Could you check a few things on this drawing? It's one solid part, dimensions in mm from its lowest x, y, z. Give positions to 0.01 mm unless a question says otherwise; leave off trailing zeros. Order: outer loops, then holes, each group sorted by start corner. A loop starts at its lowest first (then second) coordinate and runs counter-clockwise, first axis right, second up. Notation, with made-up numbers: M 65.25,6.25 L 85.25,6.25 A13 ccw 85.25,28.25 Z; hole C -23.75,42.5 d11. An arc over 180 degrees is marked long. Use one line per item in the form item = value. Start each with the question number.
1. We'd pull the mould along X, two halves only. Please class the marked faces 1, 2 and 3: +X half, -X half, draft (parallel to the pull), parting line (faces both ways), or undercut.
2. I want a section at C-C, the plane y = 2.25. List the corners of the cut face in (x, z) for me (3 decimals), and give its area (3 significant figures).
3. Will these pins go through, and if not, where does the flat tip stop? P1, Ø2, axis at x = 18.5, z = 49, coming from the -Y side; P2, Ø3, axis at x = 15, y = 4, coming from the -Z side.
4. I want a section at A-A, the plane z = 26.5. List the corners of the cut face in (x, y) for me.
5. I need wall thicknesses on L1, parallel to X at y = 1.75, z = 21.5; L2, parallel to Z at x = 12, y = 2; L3, parallel to Y at x = 14, z = 32. Which ranges of each line are inside material? Lowest first, please.
6. I want a section at B-B, the plane x = 10. List the corners of the cut face in (y, z) for me (3 decimals), and give its area (3 significant figures).
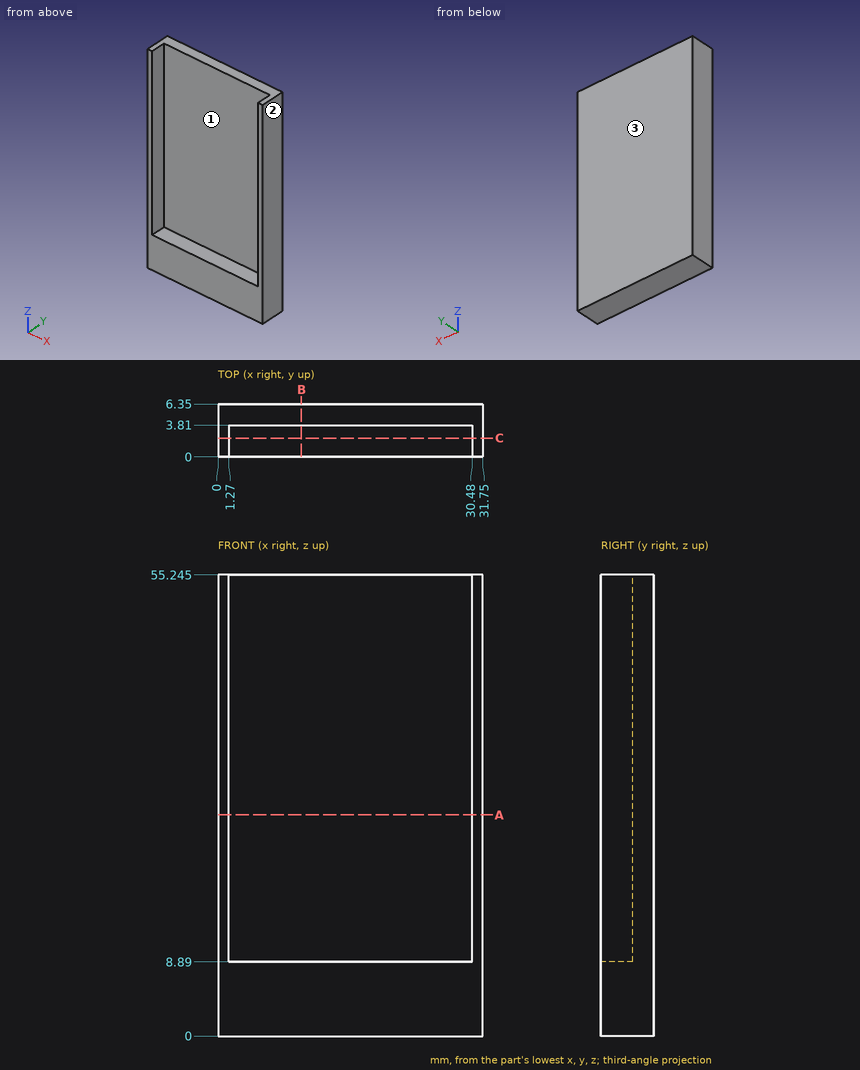
Check result:
q1.face_1 = undercut
q1.face_2 = +X half
q1.face_3 = draft
q2.outline = M 0,0 L 31.75,0 L 31.75,55.245 L 30.48,55.245 L 30.48,8.89 L 1.27,8.89 L 1.27,55.245 L 0,55.245 Z
q2.area = 400 mm2
q3.P1 = 3.81
q3.P2 = 0
q4.outline = M 0,0 L 1.27,0 L 1.27,3.81 L 30.48,3.81 L 30.48,0 L 31.75,0 L 31.75,6.35 L 0,6.35 Z
q5.L1 = 0 to 1.27, 30.48 to 31.75
q5.L2 = 0 to 8.89
q5.L3 = 3.81 to 6.35
q6.outline = M 0,0 L 6.35,0 L 6.35,55.245 L 3.81,55.245 L 3.81,8.89 L 0,8.89 Z
q6.area = 174 mm2
